Design review of the part shown in the three views and the two pictorial views. Dimensions are in mm from the part's minimum x, y and z. Coordinates: 2 decimals unless noted, no trailing zeros. Loops run counter-clockwise (first coordinate to the right, second up) from the corner with the lowest first, then second, coordinate; pieces in that order, holes last. Notation, with made-up numbers: M 79.5,35.25 L 126.5,35.25 A25 cw 126.5,74.25 Z; hole C 42.25,52 d6. An arc over 180 degrees is marked long. Answer as a JSON object with one key per item and string values. Group by question number.
Item 1: Add section A-A (z = 20). State the section outline as (x, y) points.
Item 2: Add section B-B (y = 207.5). State the section outline as (x, z) points, then the cut area to 3 significant figures.
Item 3: Wall thickness on L1, parallel to X at y = 66, z = 22.5; L2, parallel to X at y = 183, z = 33.5; L3, parallel to Z at x = 348.5, y = 147: over which ranges is each line inside the solid? List them lowest first. Write a range as from..to.
Item 4: Mouldability with a two-part tool opening along X and no side actions: class the marked faces 1, 2 and 3 as +X half, -X half, draft (parallel to the pull), parting line (faces both ways), or undercut.
Item 5: Add section C-C (x = 398.5). State the section outline as (y, z) points.
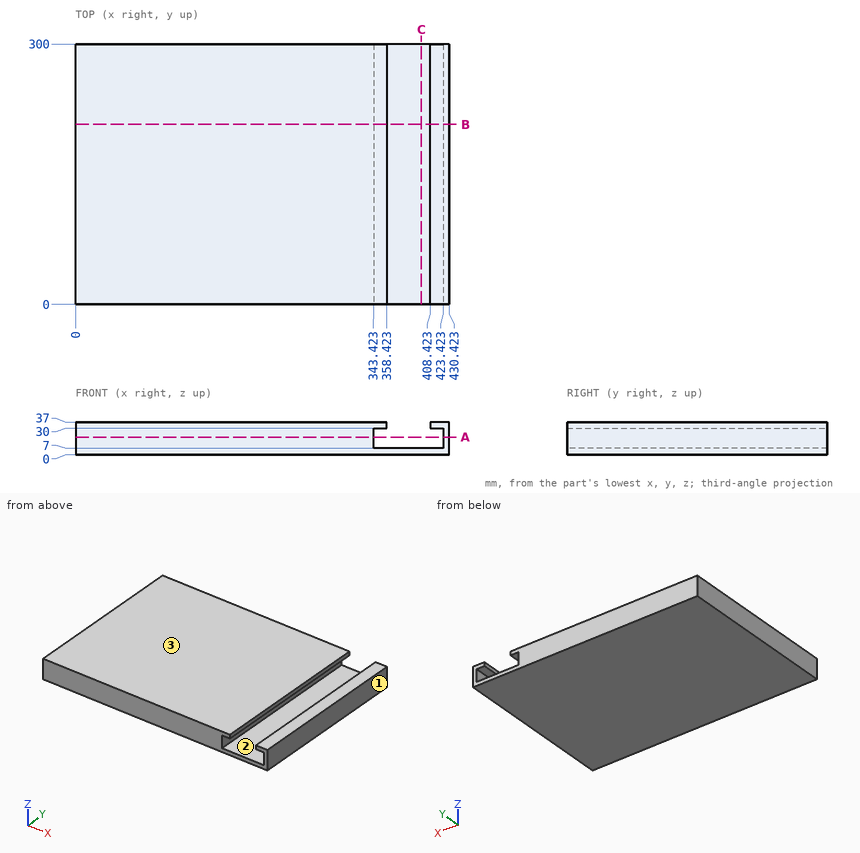
From the geometry:
{
 "1": {"outline": "M 0,0 L 343.42,0 L 343.42,300 L 0,300 Z; M 423.42,0 L 430.42,0 L 430.42,300 L 423.42,300 Z"},
 "2": {"outline": "M 0,0 L 430.42,0 L 430.42,37 L 408.42,37 L 408.42,30 L 423.42,30 L 423.42,7 L 343.42,7 L 343.42,30 L 358.42,30 L 358.42,37 L 0,37 Z", "area": "13,700 mm²"},
 "3": {"L1": "x = 0..343.42, 423.42..430.42", "L2": "x = 0..358.42, 408.42..430.42", "L3": "z = 0..7, 30..37"},
 "4": {"face 1": "+X half", "face 2": "undercut", "face 3": "draft"},
 "5": {"outline": "M 0,0 L 300,0 L 300,7 L 0,7 Z"}
}
